Part print with two shaded views. Sizes in mm from the minimum x, y, z corner. Give positions to 0.01 mm unless a question says otherwise; leave off trailing zeros. Order: outer loops, then holes, each group sorted by start corner. A loop starts at its lowest first (then second) coordinate and runs counter-clockwise, first axis right, second up. Notation, with made-up numbers: (-4.75, 84.5) -> (39.25, 84.5) arc R26 cw to (39.25, 101.5) -> close; hole circle Ø3 at (36.25, -31). An arc over 180 degrees is marked (long way). Answer in a Markdown table with one row per item. Add a question column.
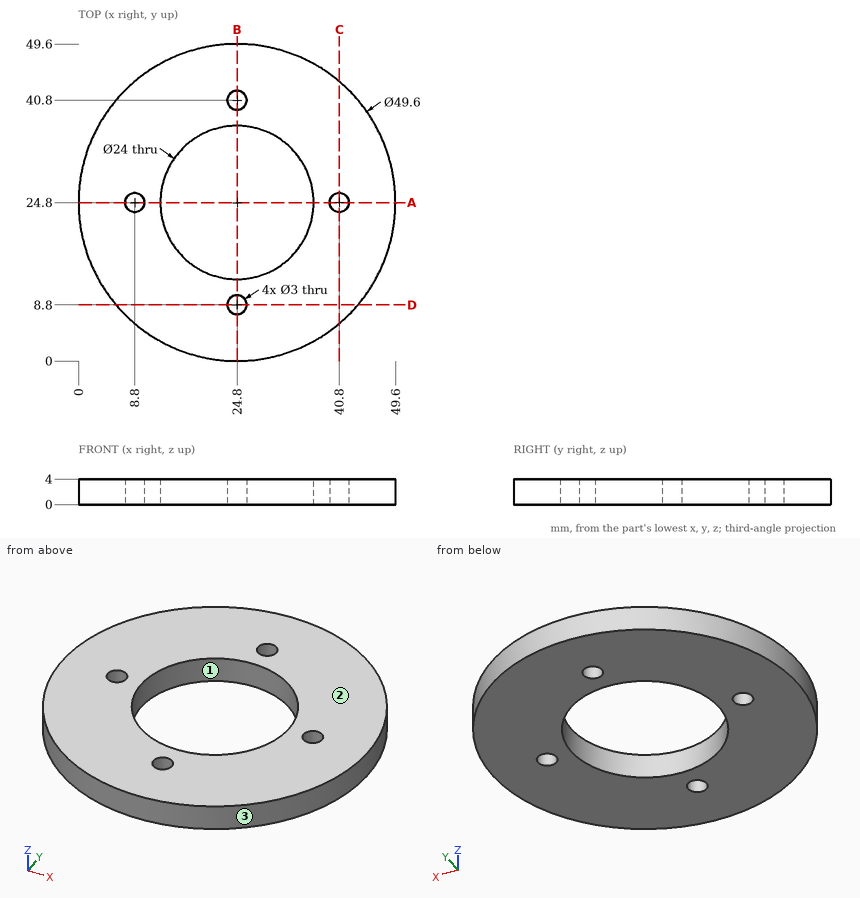
Item 1: Pin check, flat tips, straight feed: pin 1 Ø2 at (y, z) = (15.5, 2.5) entering from +X; pin 2 Ø2.5 at (x, y) = (24.8, 40.8) entering from +Z; pin 3 Ø4 at (x, y) = (8.8, 24.8) entering from +Z; pin 4 Ø2 at (x, z) = (29, 2) entering from -Y. Stop position of each tip, or through.
Item 2: Saw through at A-A on y = 24.8. List the corners of the cut face in (x, z), plus the area to 3 significant figures.
Item 3: Wall check: line 1 (Y direction, x = 24.8, z = 1.3); line 2 (X direction, y = 24, z = 2.15); line 3 (X direction, y = 23.5, z = 3.15). Give the ranges that are in metal, low to high.
Item 4: Two-plate mould, pull along Y, no slides. Class the marked faces 1, 2 and 3: pulls with the +Y half, pulls with the -Y half, needs draft (parallel to the pull), parting line crosses it, or undercut.
Item 5: Saw through at C-C on x = 40.8. List the corners of the cut face in (y, z), plus the area to 3 significant figures.
Evaluation:
| question | item | result |
|---|---|---|
| 1 | pin 1 | stops at x = 48.17 |
| 1 | pin 2 | passes through |
| 1 | pin 3 | stops at z = 4 |
| 1 | pin 4 | stops at y = 0.21 |
| 2 | outline | (0, 0) -> (7.3, 0) -> (7.3, 4) -> (0, 4) -> close; (10.3, 0) -> (12.8, 0) -> (12.8, 4) -> (10.3, 4) -> close; (36.8, 0) -> (39.3, 0) -> (39.3, 4) -> (36.8, 4) -> close; (42.3, 0) -> (49.6, 0) -> (49.6, 4) -> (42.3, 4) -> close |
| 2 | area | 78.4 mm2 |
| 3 | line 1 | y = 0 to 7.3, 10.3 to 12.8, 36.8 to 39.3, 42.3 to 49.6 |
| 3 | line 2 | x = 0.01 to 7.53, 10.07 to 12.83, 36.77 to 39.53, 42.07 to 49.59 |
| 3 | line 3 | x = 0.03 to 8.05, 9.55 to 12.87, 36.73 to 40.05, 41.55 to 49.57 |
| 4 | face 1 | undercut |
| 4 | face 2 | needs draft |
| 4 | face 3 | parting line crosses it |
| 5 | outline | (5.85, 0) -> (23.3, 0) -> (23.3, 4) -> (5.85, 4) -> close; (26.3, 0) -> (43.75, 0) -> (43.75, 4) -> (26.3, 4) -> close |
| 5 | area | 140 mm2 |
